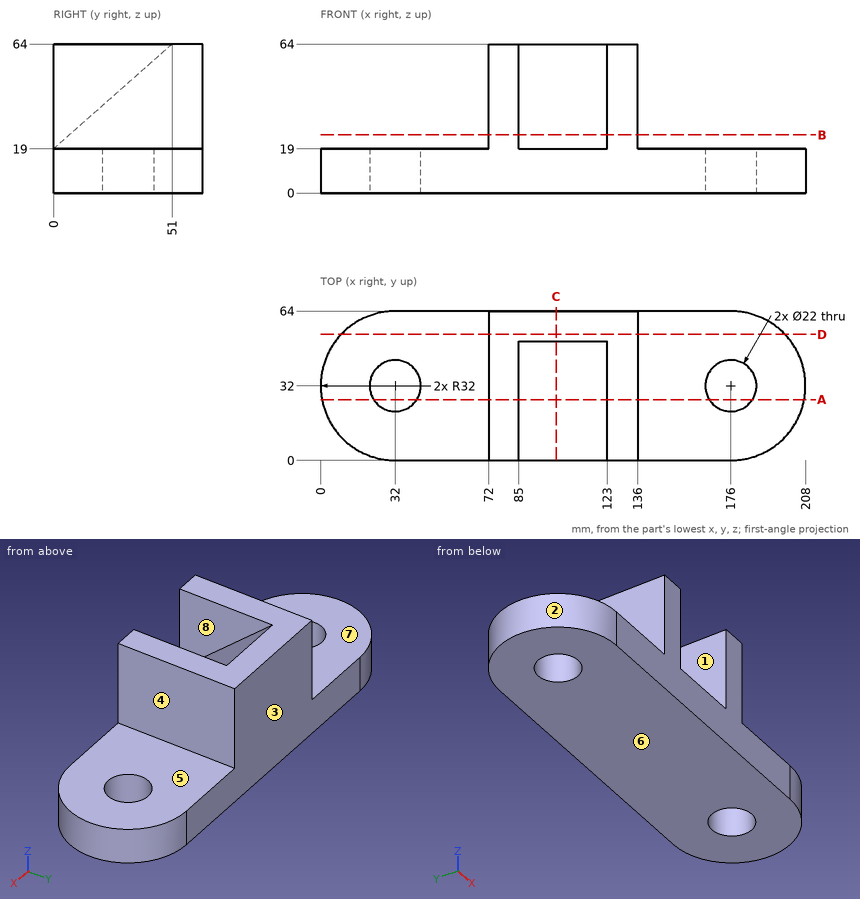
Input: dimensioned drawing with shaded views. Units: mm. Origin: part minimum x, y, z. A direction names the side the tool comes from. Round coordinates to 2 decimals unless told otherwise and drop trailing zeros. Order: outer loops, then holes, each group sorted by start corner. A loop starts at its lowest first (then second) coordinate and runs counter-clockwise, first axis right, second up. Notation, with made-up numbers: (-25.75, 75) - (6.25, 75) arc R32 ccw to (6.25, 104) - close; hole circle Ø6 at (35, 4.5). An arc over 180 degrees is marked (long way). Answer as a JSON object with one key per item and string values. Group by question number.
(1) Material intervals for probe 1 along X at (y, z) = (5, 48); probe 2 along Y at (x, z) = (32, 4.75); probe 3 along Z at (x, y) = (50.5, 7.5), sorted ascending. Write a range as from..to.
(2) Cut plane D-D (y = 54). Return loops of the section in (x, z), then the cut area to 3 significant figures.
(3) Cut plane B-B (z = 25). Return loops of the section in (x, y).
(4) Cut plane A-A (y = 26). Return loops of the section in (x, z), then the cut area to 3 significant figures.
(5) Cut plane C-C (x = 101). Return loops of the section in (y, z).
(6) Draft query along X for the marked faces 1, 2, 3 and 4. Return one class per face: released by +X, released by -X, zero draft, split by the parting line, or undercut.
(7) Reachability of the marked faces 5, 6, 7 and 8 from +Z, -Z, +X, -X, +Y, -Y: full face, straight path, thin tool, end or side. Return the list, or none.
(8) Pin query (flat end, axial travel): P1, Ø12, axis at y = 13, z = 20.5, coming from the -X side; P2, Ø10, axis at y = 26, z = 51, coming from the +X side; P3, Ø6, axis at x = 69.5, y = 39.5, coming from the -Z side; P4, Ø4, axis at y = 47.5, z = 56.5, coming from the -X side. Return the tip coordinate at first contact, or that it passes through.
Here are the results:
{
 "1": {"probe 1": "x = 72..85, 123..136", "probe 2": "y = 0..21, 43..64", "probe 3": "z = 0..19"},
 "2": {"outline": "(8.76, 0) - (199.24, 0) - (199.24, 19) - (136, 19) - (136, 64) - (72, 64) - (72, 19) - (8.76, 19) - close", "area": "6,500 mm^2"},
 "3": {"outline": "(72, 0) - (85, 0) - (85, 6.8) - (123, 6.8) - (123, 0) - (136, 0) - (136, 64) - (72, 64) - close"},
 "4": {"outline": "(0.57, 0) - (22.78, 0) - (22.78, 19) - (0.57, 19) - close; (41.22, 0) - (166.78, 0) - (166.78, 19) - (136, 19) - (136, 64) - (123, 64) - (123, 41.94) - (85, 41.94) - (85, 64) - (72, 64) - (72, 19) - (41.22, 19) - close; (185.22, 0) - (207.43, 0) - (207.43, 19) - (185.22, 19) - close", "area": "5,270 mm^2"},
 "5": {"outline": "(0, 0) - (64, 0) - (64, 64) - (51, 64) - (0, 19) - close"},
 "6": {"face 1": "undercut", "face 2": "released by -X", "face 3": "zero draft", "face 4": "released by +X"},
 "7": {"face 5": "+Z, +X, +Y, -Y", "face 6": "-Z, +X, -X, +Y, -Y", "face 7": "+Z, -X, +Y, -Y", "face 8": "+Z, -Y"},
 "8": {"P1": "stops at x = 2.85", "P2": "stops at x = 136", "P3": "stops at z = 0", "P4": "stops at x = 72"}
}
